```python
from build123d import *

# Parameters (mm, degrees)
SKETCH1_R           = 4
SKETCH1_R_2         = 1.5
BOSS_EXTRUDE1_DEPTH = 1.5
BOSS_EXTRUDE2_DEPTH = 5
SKETCH4_R           = 0.5
CUT_EXTRUDE1_DEPTH  = 14.601470509
FILLET1_R           = 1.5


with BuildPart() as part:
    # Sketch1 → Boss-Extrude1 (new body)
    with BuildSketch(Plane(origin=(0, 0, 0), x_dir=(1, 0, 0), z_dir=(0, 1, 0))):
        with Locations(Location((0, 0, 0), (0, 0, 270))):
            Circle(SKETCH1_R)
        with Locations(Location((0, 0, 0), (0, 0, 270))):
            Circle(SKETCH1_R_2, mode=Mode.SUBTRACT)
    extrude(amount=BOSS_EXTRUDE1_DEPTH)

    # Sketch3 → Boss-Extrude2 (add)
    with BuildSketch(Plane(origin=(0, 0, 0), x_dir=(1, 0, 0), z_dir=(0, 1, 0))):
        with BuildLine():
            Line((-1.5, -3.708099244), (-1.5, -6))
            Line((-1.5, -6), (1.5, -6))
            Line((1.5, -6), (1.5, -3.708099244))
            ThreePointArc((1.5, -3.708099244), (0, -4), (-1.5, -3.708099244))
        make_face()
        with BuildLine():
            Line((-1.5, 6), (1.5, 6))
            Line((1.5, 6), (1.5, 3.708099244))
            ThreePointArc((1.5, 3.708099244), (0, 4), (-1.5, 3.708099244))
            Line((-1.5, 3.708099244), (-1.5, 6))
        make_face()
    extrude(amount=BOSS_EXTRUDE2_DEPTH)

    # Sketch4 → Cut-Extrude1 (cut, through all)
    with BuildSketch(Plane.XY.offset(6)):
        with Locations((0, 3.5)):
            Circle(SKETCH4_R)
    extrude(amount=-CUT_EXTRUDE1_DEPTH, mode=Mode.SUBTRACT)

    # Fillet1
    fillet1_edges = [part.edges().sort_by_distance(p)[0] for p in [
        (1.5, 5, 4.854049622),
        (-1.5, 5, 4.854049622),
        (1.5, 5, -4.854049622),
        (-1.5, 5, -4.854049622),
    ]]
    fillet(fillet1_edges, radius=FILLET1_R - 0.0001)  # a hair under: the kernel refuses the full size


solid = part.part
```
The model under review builds one solid part; all positions refer to its coordinate system, in mm. A direction names the side the tool comes from. Round coordinates to 2 decimals unless told otherwise and drop trailing zeros. Write each loop counter-clockwise with the first axis right and the second up, starting at its lowest first coordinate (ties: lowest second). Pieces come first, ordered by that corner, then holes. Notation, with made-up numbers: (85.5, -20) - (102.5, -20) arc R11 cw to (102.5, -3) - close; hole circle Ø7 at (-2.75, -30). An arc over 180 degrees is marked (long way). Answer as CSV lines item,"result". Start each with the question number.
(1) We need section D-D on y = 3.35. State the section outline as (x, z) points, plus the area to 3 significant figures.
(2) We need section C-C on x = 1. State the section outline as (y, z) points, plus the area to 3 significant figures.
(3) We need section B-B on z = 0. State the section outline as (x, y) points, plus the area to 3 significant figures.
(4) For pin 1 Ø0.7 at (y, z) = (2, -5.5) entering from +X; pin 2 Ø1 at (y, z) = (1, -1.5) entering from -X; pin 3 Ø1.8 at (y, z) = (1, -5) entering from -X; pin 4 Ø2 at (y, z) = (2, 0.5) entering from -X, all flat-tipped, find the tip position at first contact; note any pin that passes through.
(5) We need section A-A on y = 2.8. State the section outline as (x, z) points.
(6) For faces 4 (the flat face through (1.5, 2, 5)), 5 (the flat face through (1.5, 2, -5)), 6 (the flat face through (-1.5, 2, 5)), 7 (the cylindrical face through (0, 2.8, 4)), list the 3-axis set-ups (+Z, -Z, +X, -X, +Y, -Y) from which the entire face can be reached by the end or side of a thin tool; tool diameter is ignored.
(7) To check wall thickness, follow line 1 (X direction, y = 3.5, z = -5.3); line 2 (X direction, y = 0.8, z = 0); line 3 (Z direction, x = 0, y = 2.8). State the ranges of each line that lie inside material, in increasing order.
(8) Draft analysis for pull direction Z (two halves, no side actions). For faces 1 (the cylindrical face through (-1.07, 4.55, 4.87)), 2 (the flat face through (0, 2, -6)), 3 (the cylindrical face through (0, 2.8, -4)), state which applies: pulls with the +Z half, pulls with the -Z half, needs draft (parallel to the pull), parting line crosses it, or undercut.
Worked answers:
1,outline,"(-1.5, -6) - (-0.48, -6) - (-0.48, -3.97) arc R4 cw to (-1.5, -3.71) - close; (-1.5, 3.71) arc R4 cw to (-0.48, 3.97) - (-0.48, 6) - (-1.5, 6) - close; (0.48, -6) - (1.5, -6) - (1.5, -3.71) arc R4 cw to (0.48, -3.97) - close; (0.48, 3.97) arc R4 cw to (1.5, 3.71) - (1.5, 6) - (0.48, 6) - close"
1,area,"8.74 mm²"
2,outline,"(0, -6) - (4.62, -6) - (4.62, -3.87) - (1.5, -3.87) - (1.5, -1.12) - (0, -1.12) - close; (0, 1.12) - (1.5, 1.12) - (1.5, 3.87) - (4.62, 3.87) - (4.62, 6) - (0, 6) - close"
2,area,"27.9 mm²"
3,outline,"(-4, 0) - (-1.5, 0) - (-1.5, 1.5) - (-4, 1.5) - close; (1.5, 0) - (4, 0) - (4, 1.5) - (1.5, 1.5) - close"
3,area,"7.50 mm²"
4,pin 1,"x = 1.5"
4,pin 2,"x = -3.87"
4,pin 3,"x = -1.5"
4,pin 4,"x = -4"
5,outline,"(-1.5, -6) - (1.5, -6) - (1.5, -3.71) arc R4 cw to (-1.5, -3.71) - close; (-1.5, 3.71) arc R4 cw to (1.5, 3.71) - (1.5, 6) - (-1.5, 6) - close"
6,face 4,"+Z, +X, +Y, -Y"
6,face 5,"-Z, +X, +Y, -Y"
6,face 6,"+Z, -X, +Y, -Y"
6,face 7,"+Y"
7,line 1,"-1.5 to -0.5, 0.5 to 1.5"
7,line 2,"-4 to -1.5, 1.5 to 4"
7,line 3,"-6 to -4, 4 to 6"
8,face 1,"needs draft"
8,face 2,"pulls with the -Z half"
8,face 3,"undercut"
